For this review, take the finished solid that the model builds, in its own axes (mm). Face numbers are marked on the shaded views. Coordinates: 2 decimals unless noted, no trailing zeros. Write each loop counter-clockwise with the first axis right and the second up, starting at its lowest first coordinate (ties: lowest second). Pieces come first, ordered by that corner, then holes.
```python
from build123d import *

# Parameters (mm, degrees)
F0_R     = 50
F1_DEPTH = 100
F2_T     = 5


# Not quite as in the source:
# - a fillet or chamfer that OpenCascade refuses, or shapes differently, is made with other operations: its cross-section is extruded or revolved along the edge and cut away or added
# - a feature of the source that left no trace in its solid (it failed there, or was rolled back) is left out


with BuildPart() as f1:
    # F0 (on Top) → F1 (new body)
    with BuildSketch(Plane.XY):
        Circle(F0_R)
    extrude(amount=F1_DEPTH)

    # F2
    f2_openings = [f1.faces().sort_by_distance(p)[0] for p in [
        (0, 0, 100),
    ]]
    offset(amount=F2_T, openings=f2_openings, kind=Kind.INTERSECTION)

    # F3: fillet of radius 5 on 2 edges, made by hand

    # F3_s1 → F3_t2 (revolve, cut)
    with BuildSketch(Plane.XZ):
        with BuildLine():
            ThreePointArc((50, 100), (53.5355339059, 98.5355339059), (55, 95))
            Line((55, 95), (55, 100))
            Line((55, 100), (50, 100))
        make_face()
    revolve(axis=Axis((0, 0, 100), (0, 0, -1)), mode=Mode.SUBTRACT)

    # F3_s3 → F3_t4 (revolve, cut)
    with BuildSketch(Plane.XZ):
        with BuildLine():
            ThreePointArc((55, 0), (53.5355339059, -3.5355339059), (50, -5))
            Line((50, -5), (55, -5))
            Line((55, -5), (55, 0))
        make_face()
    revolve(axis=Axis((0, 0, -5), (0, 0, -1)), mode=Mode.SUBTRACT)


solid = f1.part
```
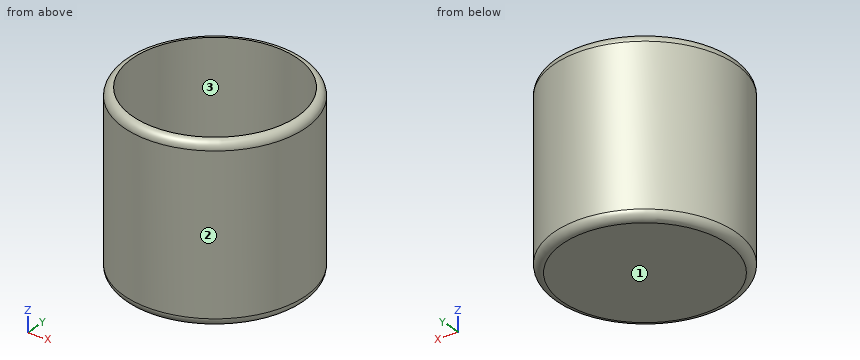
Q1. For probe 1 along Y at (x, z) = (0, 60); probe 2 along Z at (x, y) = (35, -11.5); probe 3 along X at (y, z) = (12, 1.5), list the stretches that pass through material, from the lowest coordinate up.
Ans:
probe 1: y = -55 to -50, 50 to 55
probe 2: z = -5 to 0
probe 3: x = -53.67 to -48.54, 48.54 to 53.67
Q2. Add section C-C (z = 9). State the section outline as (x, y) points, then the cut area to 3 significant figures.
Ans:
outline: circle Ø110 at (0, 0); hole circle Ø100 at (0, 0)
area: 1,650 mm2
Q3. Add section A-A (y = 0). State the section outline as (x, z) points, then the cut area to 3 significant figures.
Ans:
outline: (-55, 0) arc R5 ccw to (-50, -5) - (50, -5) arc R5 ccw to (55, 0) - (55, 95) arc R5 ccw to (50, 100) - (50, 0) - (-50, 0) - (-50, 100) arc R5 ccw to (-55, 95) - close
area: 1,530 mm2
Q4. Draft analysis for pull direction X (two halves, no side actions). For the marked faces 1, 2 and 3, state which applies: +X half, -X half, draft (parallel to the pull), parting line (faces both ways), or undercut.
Ans:
face 1: draft
face 2: parting line
face 3: undercut
Q5. Clearance check with flat-ended pins moving along their axes: pin 1 Ø8 at (y, z) = (-16, 7.5) entering from +X; pin 2 Ø8 at (x, z) = (-1.5, 43.5) entering from -Y; pin 3 Ø12 at (x, y) = (42, -20) entering from +Z; pin 4 Ø2 at (y, z) = (-30, 22.5) entering from +X. State where each tip first meets the part, or that it passes through.
Ans:
pin 1: stops at x = 53.67
pin 2: stops at y = -55
pin 3: stops at z = 100
pin 4: stops at x = 46.73
